```python
from build123d import *

# Parameters (mm, degrees)
SKETCH1_R           = 4
BOSS_EXTRUDE1_DEPTH = 25.4
SKETCH2_R           = 2.54
CUT_EXTRUDE1_DEPTH  = 39.1
SKETCH4_R           = 1.984375
CUT_EXTRUDE3_DEPTH  = 39.1
CHAMFER1_SIZE       = 1.27


with BuildPart() as part:
    # Sketch1 → Boss-Extrude1 (new body)
    with BuildSketch(Plane(origin=(0, 0, 0), x_dir=(1, 0, 0), z_dir=(0, 1, 0))):
        with BuildLine():
            Line((-3.937, 25.4), (-3.937, 8.953468099))
            ThreePointArc((-3.937, 8.953468099), (-4.340935092, 6.117132874), (-5.520621557, 3.506328226))
            ThreePointArc((-5.520621557, 3.506328226), (-4.348789534, -4.884631981), (4.121395045, -5.077962473))
            Line((4.121395045, -5.077962473), (16.637, 5.08))
            Line((16.637, 5.08), (16.637, 25.4))
            Line((16.637, 25.4), (14.097, 25.4))
            Line((14.097, 25.4), (14.097, 7.62))
            Line((14.097, 7.62), (7.747, 7.62))
            Line((7.747, 7.62), (7.747, 25.4))
            Line((7.747, 25.4), (-3.937, 25.4))
        make_face()
        with Locations(Location((0, 0, 0), (0, 0, 270))):
            Circle(SKETCH1_R, mode=Mode.SUBTRACT)
    extrude(amount=BOSS_EXTRUDE1_DEPTH)

    # Sketch2 → Cut-Extrude1 (cut, through all)
    with BuildSketch(Plane(origin=(3.937, 0, 0), x_dir=(0, 0, -1), z_dir=(1, 0, 0))):
        with Locations(Location((18.859468099, 20.32, 0), (0, 0, 180))):
            Circle(SKETCH2_R)
        with Locations(Location((18.859468099, 5.08, 0), (0, 0, 180))):
            Circle(SKETCH2_R)
    extrude(amount=CUT_EXTRUDE1_DEPTH, mode=Mode.SUBTRACT)

    # Sketch4 → Cut-Extrude3 (cut, through all)
    with BuildSketch(Plane(origin=(3.937, 0, 0), x_dir=(0, 0, -1), z_dir=(1, 0, 0))):
        with Locations((18.859468099, 20.32)):
            Circle(SKETCH4_R)
        with Locations((18.859468099, 5.08)):
            Circle(SKETCH4_R)
    extrude(amount=-CUT_EXTRUDE3_DEPTH, mode=Mode.SUBTRACT)

    # Chamfer1
    # the kernel refuses this chamfer: 1.27 mm, written as the material it adds along each edge
    with BuildSketch(Plane(origin=(3.937, 20.32, -18.859468099), x_dir=(0, 0, 1), z_dir=(0, 1, 0))) as chamfer1_piece_1_section:
        Polygon((2.54 - CHAMFER1_SIZE, 0), (2.54, CHAMFER1_SIZE), (2.54, 0), align=None)
    chamfer1_piece_1 = revolve(axis=Axis((3.937, 20.32, -18.859468099), (1, 0, 0)), mode=Mode.PRIVATE)
    chamfer1_piece_1 = chamfer1_piece_1 - Plane(origin=(4.932574819, 20.32, -18.859468099), x_dir=(0, 0, -1), z_dir=(1, 0, 0)) * Cylinder(1.984375, 11, mode=Mode.PRIVATE)
    add(chamfer1_piece_1)
    with BuildSketch(Plane(origin=(3.937, 5.08, -18.859468099), x_dir=(0, 0, 1), z_dir=(0, 1, 0))) as chamfer1_piece_2_section:
        Polygon((2.54 - CHAMFER1_SIZE, 0), (2.54, CHAMFER1_SIZE), (2.54, 0), align=None)
    chamfer1_piece_2 = revolve(axis=Axis((3.937, 5.08, -18.859468099), (1, 0, 0)), mode=Mode.PRIVATE)
    chamfer1_piece_2 = chamfer1_piece_2 - Plane(origin=(4.932574819, 5.08, -18.859468099), x_dir=(0, 0, -1), z_dir=(1, 0, 0)) * Cylinder(1.984375, 11, mode=Mode.PRIVATE)
    add(chamfer1_piece_2)


solid = part.part
```
CAD build for the part. Positions are in the model's coordinates, mm. A direction names the side the tool comes from. Round coordinates to 2 decimals unless told otherwise and drop trailing zeros. Order: outer loops, then holes, each group sorted by start corner. A loop starts at its lowest first (then second) coordinate and runs counter-clockwise, first axis right, second up.
Q1. Wall check: L1, parallel to Z at x = -0.25, y = 20.32; L2, parallel to X at y = 19.75, z = -13; L3, parallel to Z at x = -1, y = 5.08. Give the ranges that are in metal, low to high.
Q2. Slice it at A-A (y = 5.08). Write the cut outline in (x, z), and give its area (3 significant figures).
Q3. Slice it at D-D (y = 8.5). Write the cut outline in (x, z).
Q4. Drop flat-ended pins along their axis: pin 1 (5 mm diameter, centred on y = 22.5, z = -12.5, fed in from -X); pin 2 (5 mm diameter, centred on y = 20.32, z = -18.86, fed in from +X); pin 3 (3 mm diameter, centred on y = 5.08, z = -18.86, fed in from +X). Give the stop position or say it passes through.
Q5. Slice it at B-B (x = 0). Write the cut outline in (y, z), and give its area (3 significant figures).
Q6. Two-plate mould, pull along Y, no slides. Class faces 5 (the flat face through (14.097, 13, -17)), 6 (the flat face through (5, 0, -10)), 7 (the cylindrical face through (0.417, 22.287, -18.601)): pulls with the +Y half, pulls with the -Y half, needs draft (parallel to the pull), parting line crosses it, or undercut.
Q7. Which spindle directions (+Z, -Z, +X, -X, +Y, -Y) get a long thin tool onto all of the face, cutting with end or side? Do faces 1 (the cylindrical face through (15.35, 2.56, -19.19)), 2 (the flat face through (10.29, 12.52, 0.07)), 3 (the flat face through (-3.937, 13, -17)), 4 (the flat face through (7.747, 13, -16)). Say none if no direction does.
Q8. Slice it at C-C (z = -0.5). Write the cut outline in (x, y).
Results below:
1. L1: z = -25.4 to -20.84, -16.88 to -3.99, 3.99 to 6.54
1. L2: x = -3.94 to 7.75, 14.1 to 16.64
1. L3: z = -25.4 to -20.84, -16.88 to -3.87, 3.87 to 6.46
2. outline: (-5.52, -3.51) arc R10.16 cw to (-3.94, -8.95) - (-3.94, -16.88) - (4.65, -16.88) - (5.21, -16.32) - (7.75, -16.32) - (7.75, -7.62) - (14.1, -7.62) - (14.1, -16.32) - (16.64, -16.32) - (16.64, -5.08) - (4.12, 5.08) arc R6.54 ccw to start; (-3.94, -25.4) - (7.75, -25.4) - (7.75, -21.4) - (5.21, -21.4) - (4.65, -20.84) - (-3.94, -20.84) - close; (14.1, -25.4) - (16.64, -25.4) - (16.64, -21.4) - (14.1, -21.4) - close; hole circle Ø8 at (0, 0)
2. area: 366 mm2
3. outline: (-5.52, -3.51) arc R10.16 cw to (-3.94, -8.95) - (-3.94, -25.4) - (7.75, -25.4) - (7.75, -7.62) - (14.1, -7.62) - (14.1, -25.4) - (16.64, -25.4) - (16.64, -5.08) - (4.12, 5.08) arc R6.54 ccw to start; hole circle Ø8 at (0, 0)
4. pin 1: stops at x = -3.94
4. pin 2: stops at x = 5.17
4. pin 3: passes through
5. outline: (0, -25.4) - (25.4, -25.4) - (25.4, -4) - (0, -4) - close; (0, 4) - (25.4, 4) - (25.4, 6.54) - (0, 6.54) - close; hole circle Ø3.97 at (5.08, -18.86); hole circle Ø3.97 at (20.32, -18.86)
5. area: 583 mm2
6. face 5: needs draft
6. face 6: pulls with the -Y half
6. face 7: undercut
7. face 1: +X
7. face 2: +Z, +X, +Y, -Y
7. face 3: -Z, -X, +Y, -Y
7. face 4: -Z, +Y, -Y
8. outline: (-6.52, 0) - (-3.97, 0) - (-3.97, 25.4) - (-6.52, 25.4) - close; (3.97, 0) - (10.99, 0) - (10.99, 25.4) - (3.97, 25.4) - close
